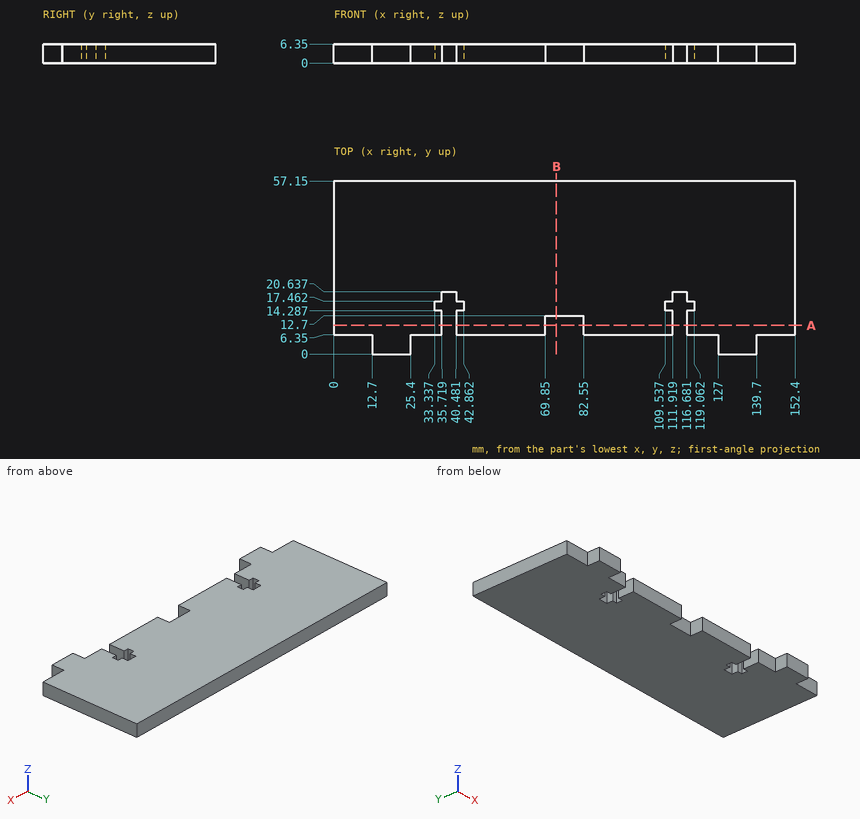
Source: three-view drawing plus pictorial views. Frame: mm from the lowest corner of the part. Give positions to 0.01 mm unless a question says otherwise; leave off trailing zeros. Loops run counter-clockwise (first coordinate to the right, second up) from the corner with the lowest first, then second, coordinate; pieces in that order, holes last.
1) Line query: L1, parallel to X at y = 10.5, z = 1; L2, parallel to Y at x = 111, z = 4.75; L3, parallel to Y at x = 121.5, z = 1.75. Output: solid intervals per line, ascending.
A:
L1: x = 0 to 35.72, 40.48 to 69.85, 82.55 to 111.92, 116.68 to 152.4
L2: y = 6.35 to 14.29, 17.46 to 57.15
L3: y = 6.35 to 57.15
2) Section query A-A on y = 9.5. Return the cut outline in (x, z).
A:
outline: (0, 0) - (35.72, 0) - (35.72, 6.35) - (0, 6.35) - close; (40.48, 0) - (69.85, 0) - (69.85, 6.35) - (40.48, 6.35) - close; (82.55, 0) - (111.92, 0) - (111.92, 6.35) - (82.55, 6.35) - close; (116.68, 0) - (152.4, 0) - (152.4, 6.35) - (116.68, 6.35) - close
3) Contact query for flat-ended pins moving along their axis: pin 1 (3 mm diameter, centred on y = 3.5, z = 4.5, fed in from -X); pin 2 (3 mm diameter, centred on x = 75, z = 2, fed in from -Y); pin 3 (2.5 mm diameter, centred on x = 37.5, z = 4.5, fed in from -Y). Output: stop coordinate, or through.
A:
pin 1: stops at x = 12.7
pin 2: stops at y = 12.7
pin 3: stops at y = 20.64
4) Section query B-B on x = 73.5. Return the cut outline in (y, z).
A:
outline: (12.7, 0) - (57.15, 0) - (57.15, 6.35) - (12.7, 6.35) - close
